For this review, take the finished solid that the model builds, in its own axes (mm). Face numbers are marked on the shaded views. A direction names the side the tool comes from. Round coordinates to 2 decimals unless told otherwise and drop trailing zeros. Order: outer loops, then holes, each group sorted by start corner. A loop starts at its lowest first (then second) coordinate and runs counter-clockwise, first axis right, second up. Notation, with made-up numbers: M 86,63.5 L 114,63.5 A11 cw 114,73.5 Z; hole C -2,2.5 d7. An arc over 180 degrees is marked long. Answer in a Markdown table with one row per item. Add a question column.
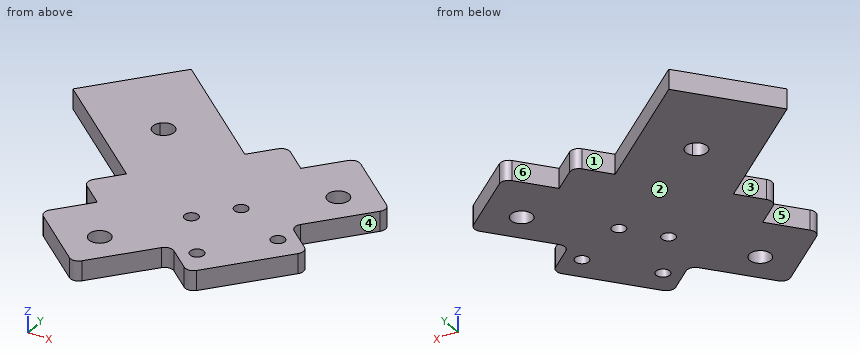
Autodesk Inventor part; units mm, degrees
ref_plane "YZ Plane" through (0, 0, 0) normal (1, 0, 0) x (0, 1, 0)
ref_plane "XZ Plane" through (0, 0, 0) normal (0, 1, 0) x (-1, 0, 0)
ref_plane "XY Plane" through (0, 0, 0) normal (0, 0, 1) x (1, 0, 0)
ref_plane "Work Plane1" through (-54.8706, 13.9436, 0) normal (0, 0, 1) x (0.7510442, -0.660252, 0)
sketch "Sketch1" plane through (-54.8706, 13.9436, 0) normal (0, 0, 1) x (0.7510442, -0.660252, 0)
  line L0 (-38.2203, 53.235) -> (-38.2203, 65.735)
  line L1 (-38.2203, 65.735) -> (-3.2203, 65.735)
  line L2 (-3.2203, 65.735) -> (-3.2203, 72.735)
  line L3 (-1.2203, 74.735) -> (5.4797, 74.735)
  line L4 (5.4797, 74.735) -> (5.4797, 84.735)
  line L5 (7.4797, 86.735) -> (24.3797, 86.735)
  line L6 (26.3797, 84.735) -> (26.3797, 67.935)
  line L7 (28.3797, 65.935) -> (35.0797, 65.935)
  line L8 (37.0797, 63.935) -> (37.0797, 53.235)
  arc A0 (37.0797, 63.935) -> (35.0797, 65.935) centre (35.0797, 63.935) ccw
  arc A1 (26.3797, 67.935) -> (28.3797, 65.935) centre (28.3797, 67.935) ccw
  arc A2 (26.3797, 84.735) -> (24.3797, 86.735) centre (24.3797, 84.735) ccw
  arc A3 (7.4797, 86.735) -> (5.4797, 84.735) centre (7.4797, 84.735) ccw
  arc A4 (-1.2203, 74.735) -> (-3.2203, 72.735) centre (-1.2203, 72.735) ccw
  circle A5 centre (30.6297, 61.785) radius 1.6
  circle A6 centre (16.7597, 58.485) radius 1.6
  circle A7 centre (18.5797, 78.435) radius 2.5
  circle A8 centre (-17.6203, 53.235) radius 2.5
  line L9 (37.0797, 53.235) -> (-15.1203, 53.235)
  line L10 (-20.1203, 53.235) -> (-38.2203, 53.235)
  point P0 (50.4165, 25.7562)
  dimension "d1" = 35
  dimension "d2" = 9
  dimension "d3" = 8.7
  dimension "d4" = 12
  dimension "d5" = 20.9
  dimension "d6" = 20.8
  dimension "d7" = 10.7
  dimension "d8" = 2
  dimension "d9" = 3.2
  dimension "d10" = 3.2
  dimension "d11" = 5
  dimension "d12" = 5
  dimension "d13" = 20.6
  dimension "d14" = 7.8
  dimension "d15" = 8.3
  dimension "d16" = 4.15
  dimension "d17" = 6.45
  dimension "d18" = 20.32
extrude "Extrusion1" add sketch "Sketch1" along normal blind 4.7 contours L0 L1 L2 A4 L3 L4 A3 L5 A2 L6 A1 L7 A0 L8 L9 A8 L10
mirror "Mirror1" about plane through (-31.078, 63.9086, 0) normal (-0.660252, -0.7510442, 0) of "Extrusion1"
properties part number "Neje_Base_Slide_y"
1. For the marked faces 4, 5 and 6, list the 3-axis set-ups (+Z, -Z, +X, -X, +Y, -Y) from which the entire face can be reached by the end or side of a thin tool; tool diameter is ignored.
2. Consider section B-B on x = -38. Write out the cut boundary in (y, z).
3. To check wall thickness, follow probe 1 along X at (y, z) = (40, 3.95); probe 2 along X at (y, z) = (70, 2.3); probe 3 along Y at (x, z) = (-35, 1.8). State the ranges of each line that lie inside material, in increasing order. Write a range as [from, to].
4. The part is to be moulded in two halves that separate along X. For the marked faces 1, 2 and 3, say which applies: pulls with the +X half, pulls with the -X half, needs draft (parallel to the pull), parting line crosses it, or undercut.
5. Consider section C-C on y = 53. Write out the cut boundary in (x, z).
6. Clearance check with a flat-ended pin moving along its axis: pin 1 Ø3 at (x, y) = (10.87, 60.58) entering from -Z. State where the tip first meets the part, or that it passes through.
Solved:
| question | item | result |
|---|---|---|
| 1 | face 4 | +Z, -Z, +X |
| 1 | face 5 | +Z, -Z, -X |
| 1 | face 6 | +Z, -Z, +Y |
| 2 | outline | M 53.35,0 L 86.64,0 L 86.64,4.7 L 53.35,4.7 Z |
| 3 | probe 1 | x = [-35.51, -11.78], [-9.42, 7.33], [10.52, 15.29] |
| 3 | probe 2 | x = [-56.48, -19.07], [-9.88, -5.44], [1.71, 12.73] |
| 3 | probe 3 | y = [22.75, 28.25], [38.75, 41.42], [50.71, 64.12], [67, 84] |
| 4 | face 1 | undercut |
| 4 | face 2 | needs draft |
| 4 | face 3 | pulls with the -X half |
| 5 | outline | M -37.6,0 L 14.59,0 L 14.59,4.7 L -37.6,4.7 Z |
| 6 | pin 1 | passes through |
